Model file for the job. Use its own axes, mm. A direction names the side the tool comes from. Give positions to 0.01 mm unless a question says otherwise; leave off trailing zeros. Loops run counter-clockwise (first coordinate to the right, second up) from the corner with the lowest first, then second, coordinate; pieces in that order, holes last. Notation, with made-up numbers: M 19,62.25 L 75,62.25 A24 cw 75,73.25 Z; hole C 29.25,4 d5. An arc over 180 degrees is marked long. Answer in a Markdown table with one row per item.
```python
from build123d import *

# Parameters (mm, degrees)
F0_W      = 22
F0_H      = 25
F1_DEPTH  = 2.5
F3_DEPTH  = 1.1
F5_DEPTH  = 25
F6_R      = 1.6
F7_DEPTH  = 29.4
F8_R      = 2.5
F9_DEPTH  = 2.5
F11_DEPTH = 2.5
F12_R     = 1
F13_SIZE  = 0.2


with BuildPart() as f1:
    # F0 (on Top) → F1 (new body, symmetric)
    with BuildSketch(Plane.XY):
        Rectangle(F0_W, F0_H)
    extrude(amount=F1_DEPTH, both=True)

    # F2 (on Top) → F3 (cut, symmetric)
    with BuildSketch(Plane.XY):
        with BuildLine():
            ThreePointArc((8.9721792225, 0), (9.180282071, 1.1164563987), (9.25, 2.25))
            ThreePointArc((9.25, 2.25), (-1.1335436013, 11.430282071), (-8.9721792225, 0))
            ThreePointArc((-8.9721792225, 0), (0, -7), (8.9721792225, 0))
        make_face()
        with BuildLine():
            ThreePointArc((8.9721792225, 0), (0, -7), (-8.9721792225, 0))
            Line((-8.9721792225, 0), (-8.9721792225, -12.5))
            Line((-8.9721792225, -12.5), (8.9721792225, -12.5))
            Line((8.9721792225, -12.5), (8.9721792225, 0))
        make_face()
    extrude(amount=F3_DEPTH, both=True, mode=Mode.SUBTRACT)

    # F4 (on Top) → F5 (cut)
    with BuildSketch(Plane.XY):
        with BuildLine():
            ThreePointArc((-6, 0), (0, -6), (6, 0))
            ThreePointArc((6, 0), (0, 6), (-6, 0))
        make_face()
        with BuildLine():
            Line((6, -12.5), (6, 0))
            ThreePointArc((6, 0), (0, -6), (-6, 0))
            Line((-6, 0), (-6, -12.5))
            Line((-6, -12.5), (6, -12.5))
        make_face()
    extrude(amount=-F5_DEPTH, mode=Mode.SUBTRACT)

    # F6 (on Top) → F7 (cut)
    with BuildSketch(Plane.XY):
        with Locations((0, -9.5)):
            Circle(F6_R)
    extrude(amount=F7_DEPTH, mode=Mode.SUBTRACT)

    # F8 (on Right) → F9 (join, symmetric)
    with BuildSketch(Plane.YZ):
        with BuildLine():
            Line((1, 9.5), (-1, 9.5))
            ThreePointArc((-1, 9.5), (-3.1213203436, 8.6213203436), (-4, 6.5))
            Line((-4, 6.5), (-4, 2.5))
            Line((-4, 2.5), (4, 2.5))
            Line((4, 2.5), (4, 6.5))
            ThreePointArc((4, 6.5), (3.1213203436, 8.6213203436), (1, 9.5))
        make_face()
        with Locations((0, 6)):
            Circle(F8_R, mode=Mode.SUBTRACT)
    extrude(amount=F9_DEPTH, both=True)

    # F10 (on Right) → F11 (join, symmetric)
    with BuildSketch(Plane.YZ):
        with BuildLine():
            ThreePointArc((4, 6.5), (3.9928498393, 6.2464249197), (4, 5.9928498393))
            Line((4, 5.9928498393), (4, 6.5))
        make_face()
        with BuildLine():
            Line((4, 2.5), (6, 2.5))
            ThreePointArc((6, 2.5), (4.5877250014, 4.0103569422), (4, 5.9928498393))
            Line((4, 5.9928498393), (4, 2.5))
        make_face()
        with BuildLine():
            ThreePointArc((-4, 5.9928498393), (-4.5877250014, 4.0103569422), (-6, 2.5))
            Line((-6, 2.5), (-4, 2.5))
            Line((-4, 2.5), (-4, 5.9928498393))
        make_face()
        with BuildLine():
            Line((-4, 6.5), (-4, 5.9928498393))
            ThreePointArc((-4, 5.9928498393), (-3.9928498393, 6.2464249197), (-4, 6.5))
        make_face()
    extrude(amount=F11_DEPTH, both=True)

    # F12
    f12_edges = [f1.edges().sort_by_distance(p)[0] for p in [
        (-11, 0, -2.5),
        (-11, 0, 2.5),
        (11, 0, 2.5),
        (11, 0, -2.5),
        (0, -12.5, 2.5),
        (0, 12.5, 2.5),
        (0, 12.5, -2.5),
        (8.5, -12.5, -2.5),
        (-8.5, -12.5, -2.5),
        (6, -6.25, -2.5),
    ]]
    fillet(f12_edges, radius=F12_R)

    # F13
    f13_edges = [f1.edges().sort_by_distance(p)[0] for p in [
        (2.5, -2.5, 6),
        (-2.5, -2.5, 6),
    ]]
    chamfer(f13_edges, length=F13_SIZE)


solid = f1.part
```
Q1. Saw through at B-B (z = 0.75). Give the cut face in (x, y).
Reported:
| item | result |
|---|---|
| outline | M -11,-12.5 L -8.97,-12.5 L -8.97,0 A9.25 cw long 8.97,0 L 8.97,-12.5 L 11,-12.5 L 11,12.5 L -11,12.5 Z |
Q2. 3-axis set-ups, long thin cutter, end or side, ignore diameter. For faces 5 (the face through (0.1, 6, -1.3)), 6 (the face through (2.5, 0, 3)), 7 (the face through (-8.972, -6, 0)), 8 (the face through (0.04, -3.1, 8.64)), 9 (the face through (-0.03, -0.33, 8.48)): which of +Z, -Z, +X, -X, +Y, -Y reach the whole face in a straight line?
Reported:
| item | result |
|---|---|
| face 5 | -Z, -Y |
| face 6 | +Z, +X, +Y, -Y |
| face 7 | -Y |
| face 8 | +Z, +X, -X, -Y |
| face 9 | +X, -X |
Q3. Mould opens along Z. For faces 1 (the face through (8.972, -6, 0)), 2 (the face through (0.154, -12.199, 2.215)), 3 (the face through (0.154, 12.199, -2.215)), 4 (the face through (0, 12.5, 0)) say: released by +Z, released by -Z, zero draft, split by the parting line, or undercut.
Reported:
| item | result |
|---|---|
| face 1 | undercut |
| face 2 | released by +Z |
| face 3 | released by -Z |
| face 4 | zero draft |
Q4. Saw through at C-C (y = -9.5). Give the cut face in (x, z), and give its area (3 significant figures).
Reported:
| item | result |
|---|---|
| outline | M -11,-1.5 A1 ccw -10,-2.5 L -7,-2.5 A1 ccw -6,-1.5 L -6,-1.1 L -8.97,-1.1 L -8.97,1.1 L -1.6,1.1 L -1.6,2.5 L -10,2.5 A1 ccw -11,1.5 Z; M 1.6,1.1 L 8.97,1.1 L 8.97,-1.1 L 6,-1.1 L 6,-1.5 A1 ccw 7,-2.5 L 10,-2.5 A1 ccw 11,-1.5 L 11,1.5 A1 ccw 10,2.5 L 1.6,2.5 Z |
| area | 48.0 mm² |
Q5. Probe probe 1 along Z at (x, y) = (1, 0); probe 2 along Z at (x, y) = (-7, -0.75); probe 3 along Y at (x, z) = (0, 1.55). List the from-to ranges inside material, lowest first.
Reported:
| item | result |
|---|---|
| probe 1 | 1.1 to 3.5, 8.5 to 9.5 |
| probe 2 | -2.5 to -1.1, 1.1 to 2.5 |
| probe 3 | -12.5 to -11.1, -7.9 to 12.5 |
Q6. Saw through at A-A (x = 0). Give the cut face in (y, z), and give its area (3 significant figures).
Reported:
| item | result |
|---|---|
| outline | M -12.5,1.1 L -11.1,1.1 L -11.1,2.5 L -11.5,2.5 A1 ccw -12.5,1.5 Z; M -7.9,1.1 L 11.5,1.1 L 11.5,-1.1 L 6,-1.1 L 6,-1.5 A1 ccw 7,-2.5 L 11.5,-2.5 A1 ccw 12.5,-1.5 L 12.5,1.5 A1 ccw 11.5,2.5 L 6,2.5 A4.5 cw 4,5.99 L 4,6.5 A3 ccw 1,9.5 L -1,9.5 A3 ccw -4,6.5 L -4,5.99 A4.5 cw -6,2.5 L -7.9,2.5 Z; hole C 0,6 d5 |
| area | 77.9 mm² |
Q7. Drop flat-ended pins along their axis: pin 1 (4.5 mm diameter, centred on y = 0, z = 6, fed in from +X); pin 2 (3.5 mm diameter, centred on x = 0, y = -9.5, fed in from -Z); pin 3 (3 mm diameter, centred on x = 0, z = 7.5, fed in from -Y); pin 4 (3.5 mm diameter, centred on y = -2.5, z = 6, fed in from +X). Give the stop position or say it passes through.
Reported:
| item | result |
|---|---|
| pin 1 | through |
| pin 2 | z = 1.1 |
| pin 3 | y = -4 |
| pin 4 | x = 2.5 |
